Input: part model. Units: mm. Frame: model coordinates. Round coordinates to 2 decimals unless told otherwise and drop trailing zeros. Loops run counter-clockwise (first coordinate to the right, second up) from the corner with the lowest first, then second, coordinate; pieces in that order, holes last. Notation, with made-up numbers: M 18.5,8 L 45.5,8 A21 cw 45.5,36 Z; hole C 80.25,29 d1. An arc over 180 degrees is marked long. Put each result on its own line as item: value. Start each with the question number.
1) Section B-B on x = 154. Output: boundary loops of the cut face in (y, z) (3 decimals).
2) Line query: probe 1 along Y at (x, z) = (122, 6.25); probe 2 along X at (y, z) = (559, 22.5); probe 3 along Y at (x, z) = (1184, 15.25). Output: solid intervals per line, ascending.
3) Section D-D on y = -308. Output: boundary loops of the cut face in (x, z) (3 decimals).
4) Pin query (flat end, axial travel): pin 1 (14.5 mm diameter, centred on y = -25.5, z = 15, fed in from +X). Return the tip coordinate at first contact, or that it passes through.
5) Section A-A on z = 8. Output: boundary loops of the cut face in (x, y), plus the area to 3 significant figures.
6) Section C-C on y = 464. Output: boundary loops of the cut face in (x, z) (3 decimals), plus the area to 3 significant figures.
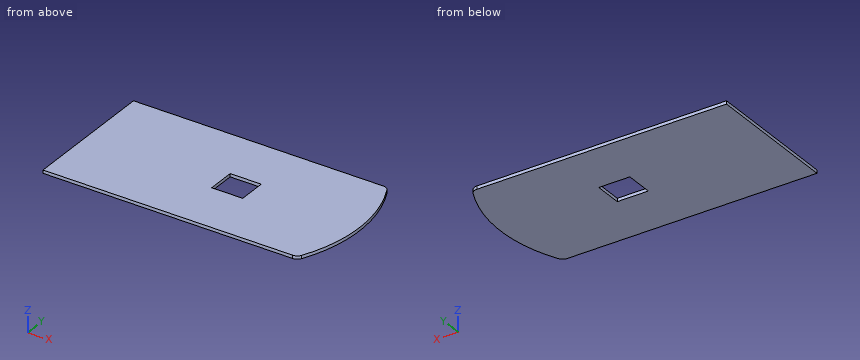
from build123d import *

# Parameters (mm, degrees)
F1_DEPTH = 28.575


# Not quite as in the source:
# - a feature names something its author has since deleted; it is built from what else it names


with BuildPart() as f1:
    # F0 (on Top) → F1 (new body)
    with BuildSketch(Plane.XY):
        with BuildLine():
            Line((1104.2429080596, 609.6), (-1143, 609.6))
            Line((-1143, 609.6), (-1143, 0))
            Line((-1143, 0), (50.8, 0))
            Line((50.8, 0), (50.8, 124.587))
            Line((50.8, 124.587), (330.2, 124.587))
            Line((330.2, 124.587), (330.2, 0))
            Line((330.2, 0), (1143, 0))
            Line((1143, 0), (1295.4, 0))
            ThreePointArc((1295.4, 0), (1261.3943180258, 294.8652818701), (1161.1626455885, 574.2494845361))
            ThreePointArc((1161.1626455885, 574.2494845361), (1137.7448313773, 600.0432213908), (1104.2429080596, 609.6))
        make_face()
        with BuildLine():
            Line((50.8, 0), (-1143, 0))
            Line((-1143, 0), (-1143, -609.6))
            Line((-1143, -609.6), (1104.2429080596, -609.6))
            ThreePointArc((1104.2429080596, -609.6), (1137.7448313773, -600.0432213908), (1161.1626455885, -574.2494845361))
            ThreePointArc((1161.1626455885, -574.2494845361), (1261.3943180258, -294.8652818701), (1295.4, 0))
            Line((1295.4, 0), (1143, 0))
            Line((1143, 0), (330.2, 0))
            Line((330.2, 0), (330.2, -124.587))
            Line((330.2, -124.587), (50.8, -124.587))
            Line((50.8, -124.587), (50.8, 0))
        make_face()
    extrude(amount=F1_DEPTH)


solid = f1.part
Geometry results:
1. outline: M -609.6,0 L -124.587,0 L -124.587,28.575 L -609.6,28.575 Z; M 124.587,0 L 609.6,0 L 609.6,28.575 L 124.587,28.575 Z
2. probe 1: y = -609.6 to -124.59, 124.59 to 609.6
2. probe 2: x = -1143 to 1168.58
2. probe 3: y = -525.55 to 525.55
3. outline: M -1143,0 L 1258.252,0 L 1258.252,28.575 L -1143,28.575 Z
4. pin 1: stops at x = 1295.27
5. outline: M -1143,-609.6 L 1104.24,-609.6 A63.5 ccw 1161.16,-574.25 A1295.4 ccw 1161.16,574.25 A63.5 ccw 1104.24,609.6 L -1143,609.6 Z; hole M 50.8,-124.59 L 330.2,-124.59 L 330.2,124.59 L 50.8,124.59 Z
5. area: 2,840,000 mm²
6. outline: M -1143,0 L 1209.448,0 L 1209.448,28.575 L -1143,28.575 Z
6. area: 67,200 mm²
